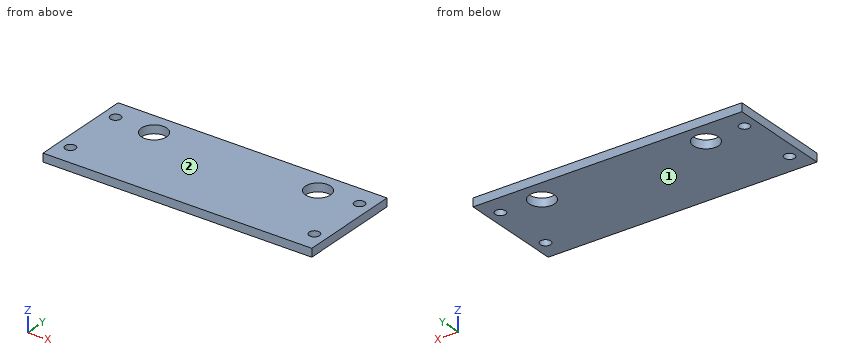
from build123d import *

# Parameters (mm, degrees)
SKETCH_1_W      = 65
SKETCH_1_H      = 25
SKETCH_1_R      = 3.05
EXTRUDE_1_DEPTH = 2
M3X0_5_1_D      = 2.5
M3X0_5_1_DEPTH  = 8.5
M3X0_5_1_TIP    = 0.751075774


with BuildPart() as part:
    # ｽｹｯﾁ1 → ﾎﾞｽ - 押し出し1 (new body)
    with BuildSketch(Plane.XY):
        Rectangle(SKETCH_1_W, SKETCH_1_H)
        with Locations((-19.83, 7)):
            Circle(SKETCH_1_R, mode=Mode.SUBTRACT)
        with Locations((19.83, 7)):
            Circle(SKETCH_1_R, mode=Mode.SUBTRACT)
    extrude(amount=EXTRUDE_1_DEPTH)

    # M3x0.5 ねじ穴1
    with Locations(Plane(origin=(-29.5, 7.5, 2), x_dir=(1, 0, 0), z_dir=(0, 0, 1))):
        with Locations((0, 0), (0, -15), (59, 0), (59, -15)):
            Hole(M3X0_5_1_D / 2, depth=M3X0_5_1_DEPTH)
            with Locations((0, 0, -(M3X0_5_1_DEPTH + M3X0_5_1_TIP / 2))):  # 118° drill point
                Cone(0, M3X0_5_1_D / 2, M3X0_5_1_TIP, mode=Mode.SUBTRACT)


solid = part.part
Geometry: final body of the model. Coordinates: model frame, mm. Face numbers are marked on the shaded views. Coordinates: 2 decimals unless noted, no trailing zeros. Loops run counter-clockwise (first coordinate to the right, second up) from the corner with the lowest first, then second, coordinate; pieces in that order, holes last. Notation, with made-up numbers: (-20.75, 47) - (25.25, 47) arc R27 ccw to (25.25, 78) - close; hole circle Ø10 at (44.5, 70.25). An arc over 180 degrees is marked (long way). Put each result on its own line as item: value. Start each with the question number.
Q1. Line query: line 1 (Y direction, x = 29.5, z = 1.35); line 2 (X direction, y = -7.75, z = 0.45); line 3 (Y direction, x = -19.83, z = 1.3). Output: solid intervals per line, ascending.
Q2. Cut plane D-D, the plane x = -19.83. Return loops of the section in (y, z).
Q3. Cut plane A-A, the plane z = 0.85. Return loops of the section in (x, y).
Q4. Pull-direction query (Z, two-part tool) for the marked faces 1 and 2; classes: released by +Z, released by -Z, zero draft, split by the parting line, or undercut.
Q5. Cut plane C-C, the plane y = -7.5. Return loops of the section in (x, z).
Q6. Cut plane B-B, the plane x = -29.5. Return loops of the section in (y, z), and give its area (3 significant figures).
Filled sheet:
1. line 1: -12.5 to -8.75, -6.25 to 6.25, 8.75 to 12.5
1. line 2: -32.5 to -30.72, -28.28 to 28.28, 30.72 to 32.5
1. line 3: -12.5 to 3.95, 10.05 to 12.5
2. outline: (-12.5, 0) - (3.95, 0) - (3.95, 2) - (-12.5, 2) - close; (10.05, 0) - (12.5, 0) - (12.5, 2) - (10.05, 2) - close
3. outline: (-32.5, -12.5) - (32.5, -12.5) - (32.5, 12.5) - (-32.5, 12.5) - close; hole circle Ø2.5 at (-29.5, -7.5); hole circle Ø2.5 at (-29.5, 7.5); hole circle Ø6.1 at (-19.83, 7); hole circle Ø6.1 at (19.83, 7); hole circle Ø2.5 at (29.5, -7.5); hole circle Ø2.5 at (29.5, 7.5)
4. face 1: released by -Z
4. face 2: released by +Z
5. outline: (-32.5, 0) - (-30.75, 0) - (-30.75, 2) - (-32.5, 2) - close; (-28.25, 0) - (28.25, 0) - (28.25, 2) - (-28.25, 2) - close; (30.75, 0) - (32.5, 0) - (32.5, 2) - (30.75, 2) - close
6. outline: (-12.5, 0) - (-8.75, 0) - (-8.75, 2) - (-12.5, 2) - close; (-6.25, 0) - (6.25, 0) - (6.25, 2) - (-6.25, 2) - close; (8.75, 0) - (12.5, 0) - (12.5, 2) - (8.75, 2) - close
6. area: 40.0 mm²
